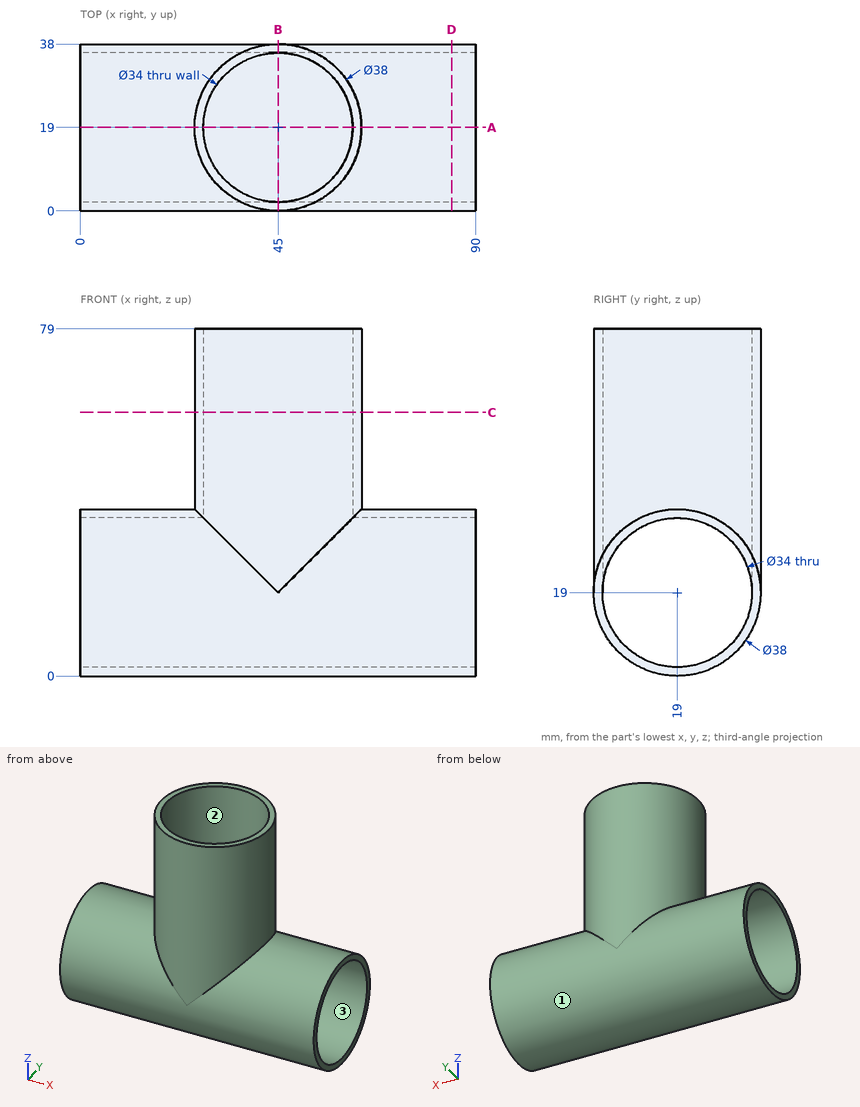
Answer from the drawing. Dimensions are ordinates in mm from the lowest x, y and z of the part. Round coordinates to 2 decimals unless told otherwise and drop trailing zeros. Write each loop counter-clockwise with the first axis right and the second up, starting at its lowest first coordinate (ties: lowest second). Pieces come first, ordered by that corner, then holes. Notation, with made-up numbers: M 0.5,89.5 L 7.5,89.5 A27 cw 7.5,115.5 Z; hole C 73,-8 d7. An arc over 180 degrees is marked long. One line per item, written item: value.
Q1. Find section A-A on y = 19. Write down the section's boundary in (x, z).
Data:
outline: M 0,0 L 90,0 L 90,2 L 0,2 Z; M 0,36 L 28,36 L 28,79 L 26,79 L 26,38 L 0,38 Z; M 62,36 L 90,36 L 90,38 L 64,38 L 64,79 L 62,79 Z
Q2. Flat-ended cylindrical pins translate along their axes: pin 1 Ø4 at (x, y) = (59, 14.5) entering from -Z; pin 2 Ø3 at (x, y) = (13, 5.5) entering from -Z; pin 3 Ø3 at (y, z) = (25.5, 45.5) entering from -X. Find the tip coordinate at first contact, or state that the pin passes through.
Data:
pin 1: z = 0.17
pin 2: z = 4.27
pin 3: x = 26.67
Q3. Find section B-B on x = 45. Write down the section's boundary in (y, z).
Data:
outline: M 0,19 A19 ccw 38,19 L 38,79 L 36,79 L 36,19 A17 cw 2,19 L 2,79 L 0,79 Z
Q4. Find section C-C on z = 60. Write down the section's boundary in (x, y).
Data:
outline: C 45,19 d38; hole C 45,19 d34
Q5. Straight lines are drawn through the part: line 1 (X direction, y = 19, z = 50); line 2 (Z direction, x = 66.5, y = 19.5); line 3 (Y direction, x = 29, z = 19). For each, find the intervals that lie inside material, in ascending order. Write a range as [from, to].
Data:
line 1: [26, 28], [62, 64]
line 2: [0.01, 2.01], [35.99, 37.99]
line 3: [0, 2], [36, 38]
Q6. For a pull along Z with two mould halves and no side action, classify the marked faces 1, 2 and 3 as +Z half, -Z half, draft (parallel to the pull), parting line (faces both ways), or undercut.
Data:
face 1: parting line
face 2: draft
face 3: undercut
Q7. Find section D-D on x = 84.5. Write down the section's boundary in (y, z).
Data:
outline: C 19,19 d38; hole C 19,19 d34
